Source: CAD feature listing. Evaluate the final solid. Frame: model axes, mm. A direction names the side the tool comes from. Coordinates: 2 decimals unless noted, no trailing zeros. Order: outer loops, then holes, each group sorted by start corner. A loop starts at its lowest first (then second) coordinate and runs counter-clockwise, first axis right, second up.
```python
from build123d import *

# Parameters (mm, degrees)
SKETCH005_R     = 0.8
PAD001_DEPTH    = 0.6
SKETCH006_R     = 3
PAD002_DEPTH    = 6.4
SKETCH007_R     = 1.8
POCKET003_DEPTH = 9
CHAMFER_SIZE    = 0.2


with BuildPart() as part:
    # Sketch005 → Pad001 (new body)
    with BuildSketch(Plane.XZ):
        with BuildLine():
            Line((7.2, 7.6), (0, 7.6))
            Line((0, 7.6), (0, 0))
            Line((0, 0), (2.5, 0))
            Line((2.5, 0), (2.5, -4.8))
            ThreePointArc((2.5, -4.8), (3.6, -5.9), (4.7, -4.8))
            Line((4.7, -4.8), (4.7, 0))
            Line((4.7, 0), (7.2, 0))
            Line((7.2, 0), (7.2, 7.6))
        make_face()
        with Locations((3.6, -4.8)):
            Circle(SKETCH005_R, mode=Mode.SUBTRACT)
    extrude(amount=PAD001_DEPTH)

    # Sketch006 (on Face11 of Pad001) → Pad002 (join)
    with BuildSketch(Plane.XZ.offset(0.6)):
        with Locations((3.6, 4.1)):
            Circle(SKETCH006_R)
    extrude(amount=PAD002_DEPTH)

    # Sketch007 (on Face13 of Pad002) → Pocket003 (cut)
    with BuildSketch(Plane.XZ.offset(7)):
        with Locations((3.6, 4.1)):
            Circle(SKETCH007_R)
    extrude(amount=-POCKET003_DEPTH, mode=Mode.SUBTRACT)

    # Chamfer
    chamfer_edges = [part.edges().sort_by_distance(p)[0] for p in [
        (0.6, -7, 4.1),
        (1.8, -7, 4.1),
    ]]
    chamfer(chamfer_edges, length=CHAMFER_SIZE)


with BuildPart() as part_1:
    # Body placement: moved
    add(part.part.moved(Location((1.4, 2.6, 1.4))))


solid = part_1.part
```
Q1. Section query B-B on x = 5. Output: boundary loops of the cut face in (y, z).
Solutions:
outline: (-4.4, 2.7) - (-4.2, 2.5) - (2, 2.5) - (2, -2.6) - (2.6, -2.6) - (2.6, 3.7) - (-4.2, 3.7) - (-4.4, 3.5) - close; (-4.4, 7.5) - (-4.2, 7.3) - (2.6, 7.3) - (2.6, 9) - (2, 9) - (2, 8.5) - (-4.2, 8.5) - (-4.4, 8.3) - close; (2, -4.5) - (2.6, -4.5) - (2.6, -4.2) - (2, -4.2) - close
Q2. Section query D-D on z = -0.5. Output: boundary loops of the cut face in (x, y), plus the area to 3 significant figures.
Solutions:
outline: (3.9, 2) - (6.1, 2) - (6.1, 2.6) - (3.9, 2.6) - close
area: 1.32 mm2
Q3. Set-up query: faces 5 (the flat face through (7, -4.4, 4)), 6 (the cylindrical face through (4.35, -1.06, 2.57)). Return all of +Z, -Z, +X, -X, +Y, -Y with unobstructed straight access to the full face (end or side cutting, diameter ignored); none if empty.
Solutions:
face 5: +Z, -Z, +X, -X, -Y
face 6: -Y
Q4. Section query C-C on y = 1. Output: boundary loops of the cut face in (x, z).
Solutions:
outline: circle Ø6 at (5, 5.5); hole circle Ø3.6 at (5, 5.5)
Q5. Section query A-A on z = 5.5. Output: boundary loops of the cut face in (x, y).
Solutions:
outline: (1.4, 2) - (2, 2) - (2, -4.2) - (2.2, -4.4) - (3, -4.4) - (3.2, -4.2) - (3.2, 2.6) - (1.4, 2.6) - close; (6.8, -4.2) - (7, -4.4) - (7.8, -4.4) - (8, -4.2) - (8, 2) - (8.6, 2) - (8.6, 2.6) - (6.8, 2.6) - close
Q6. Material intervals for line 1 along Z through (x, y) = (5, 2.3); line 2 along Z through (x, y) = (5, -1.75); line 3 along Z through (x, y) = (4.5, 2.25), sorted ascending.
Solutions:
line 1: z = -4.5 to -4.2, -2.6 to 3.7, 7.3 to 9
line 2: z = 2.5 to 3.7, 7.3 to 8.5
line 3: z = -4.38 to -4.02, -2.78 to 3.77, 7.23 to 9
Q7. Pull-direction query (X, two-part tool) for faces 1 (the flat face through (5, 2.6, 2)), 2 (the cylindrical face through (4.2, 2.3, -3.4)), 3 (the cylindrical face through (5, 2.3, -4.5)), 4 (the cylindrical face through (5.831, -0.848, 3.903)); classes: pulls with the +X half, pulls with the -X half, needs draft (parallel to the pull), parting line crosses it, or undercut.
Solutions:
face 1: needs draft
face 2: undercut
face 3: parting line crosses it
face 4: undercut
Q8. Pin query (flat end, axial travel): P1, Ø0.7, axis at x = 3, y = 2, coming from the -Z side; P2, Ø2.5, axis at x = 5, z = -3.4, coming from the -Y side. Return the tip coordinate at first contact, or that it passes through.
Solutions:
P1: stops at z = 1.4
P2: stops at y = 2
